Design review of the part built by this model. Coordinates are the model's own, in mm. A direction names the side the tool comes from. Round coordinates to 2 decimals unless told otherwise and drop trailing zeros. Write each loop counter-clockwise with the first axis right and the second up, starting at its lowest first coordinate (ties: lowest second). Pieces come first, ordered by that corner, then holes. Notation, with made-up numbers: (40, 65.25) -> (73, 65.25) arc R33 ccw to (73, 103.25) -> close; hole circle Ø7 at (74, 41.5). An arc over 180 degrees is marked (long way). Write item = value, one per line. Start each with the question number.
Item 1: For pin 1 Ø3 at (x, y) = (116, -31) entering from +Z; pin 2 Ø3 at (x, y) = (48, -29) entering from +Z; pin 3 Ø8 at (x, y) = (21, -20) entering from -Z, all flat-tipped, find the tip position at first contact; note any pin that passes through.
Item 2: Machinability: for faces 4 (the flat face through (48, -18, 6)), 5 (the flat face through (122, -27.059, 4)), 6 (the flat face through (50, -27.3, 4.5)), 7 (the flat face through (109, -30, 6)), 8 (the flat face through (3, -13, -13)), which of the approach directions +Z, -Z, +X, -X, +Y, -Y give a long, thin tool a straight path to every point of the face, cutting with its end or side? Answer none if there is none.
Item 3: Add section C-C, the plane x = 134.5. State the section outline as (y, z) points.
Item 4: Mouldability with a two-part tool opening along X and no side actions: class faces 1 (the flat face through (0, -13, -9)), 2 (the flat face through (113, -30, 5)), 3 (the flat face through (5, -23, 10)) as released by +X, released by -X, zero draft, split by the parting line, or undercut.
Item 5: Add section D-D, the plane y = -3. State the section outline as (x, z) points.
Item 6: Add section A-A, the plane y = -21. State the section outline as (x, z) points.
Item 7: To check wall thickness, follow L1, parallel to Z at x = 110.5, y = -30; L2, parallel to X at y = -17, z = -5; L3, parallel to Z at x = 68.5, y = -28.5. State the ranges of each line that lie inside material, in increasing order.
Item 8: Add section B-B, the plane z = 6.25. State how many separate pieces and enclosed holes the cut face has, then the cut area to 3 significant figures.
from build123d import *

# Parameters (mm, degrees)
SKETCH1_W           = 3
SKETCH1_H           = 20
BOSS_EXTRUDE1_DEPTH = 140
SKETCH3_W           = 10
SKETCH3_H           = 5.940571325
SKETCH3_W_2         = 4
SKETCH3_W_3         = 35
BOSS_EXTRUDE2_DEPTH = 10
SKETCH5_W           = 38
SKETCH5_H           = 5
CUT_EXTRUDE2_DEPTH  = 15
SKETCH6_W           = 10
SKETCH6_H           = 2.5
SKETCH6_W_2         = 4
BOSS_EXTRUDE4_DEPTH = 15
SKETCH7_R           = 1.75
SKETCH7_W           = 7.5
SKETCH7_H           = 2.5
CUT_EXTRUDE3_DEPTH  = 15
SKETCH9_W           = 20
SKETCH9_H           = 40
SKETCH9_R           = 2.25
BOSS_EXTRUDE5_DEPTH = 3
BOSS_EXTRUDE6_DEPTH = 3


with BuildPart() as part:
    # Sketch1 → Boss-Extrude1 (new body)
    with BuildSketch(Plane(origin=(0, 0, 0), x_dir=(0, 0, -1), z_dir=(1, 0, 0))):
        with Locations((1.5, -23)):
            Rectangle(SKETCH1_W, SKETCH1_H)
    extrude(amount=BOSS_EXTRUDE1_DEPTH)

    # Sketch3 → Boss-Extrude2 (add)
    with BuildSketch(Plane.XY):
        with Locations((5, -30.029714338)):
            Rectangle(SKETCH3_W, SKETCH3_H)
        with Locations((48, -30.029714338)):
            Rectangle(SKETCH3_W_2, SKETCH3_H)
        with Locations((82, -30.029714338)):
            Rectangle(SKETCH3_W_2, SKETCH3_H)
        with Locations((122.5, -30.029714338)):
            Rectangle(SKETCH3_W_3, SKETCH3_H)
    extrude(amount=BOSS_EXTRUDE2_DEPTH)

    # Sketch5 → Cut-Extrude2 (cut)
    with BuildSketch(Plane.XZ.offset(33)):
        with Locations((65, 7.5)):
            Rectangle(SKETCH5_W, SKETCH5_H)
    extrude(amount=-CUT_EXTRUDE2_DEPTH, mode=Mode.SUBTRACT)

    # Sketch6 → Boss-Extrude4 (add)
    with BuildSketch(Plane.XZ.offset(33)):
        with Locations((5, 11.25)):
            Rectangle(SKETCH6_W, SKETCH6_H)
        with Locations((48, 6.25)):
            Rectangle(SKETCH6_W_2, SKETCH6_H)
        with Locations((82, 6.25)):
            Rectangle(SKETCH6_W_2, SKETCH6_H)
    extrude(amount=-BOSS_EXTRUDE4_DEPTH)

    # Sketch7 → Cut-Extrude3 (cut)
    with BuildSketch(Plane(origin=(0, -27.059428675, 0), x_dir=(1, 0, 0), z_dir=(0, 1, 0))):
        with Locations((128.5, -6.25)):
            Circle(SKETCH7_R)
        with Locations((122.5, -6.25)):
            Circle(SKETCH7_R)
        with Locations((134.5, -6.25)):
            Circle(SKETCH7_R)
        with Locations((112.75, -6.25)):
            Rectangle(SKETCH7_W, SKETCH7_H)
    extrude(amount=-CUT_EXTRUDE3_DEPTH, mode=Mode.SUBTRACT)

    # Sketch9 → Boss-Extrude5 (add)
    with BuildSketch(Plane.ZY):
        with Locations((-13, -13)):
            Rectangle(SKETCH9_W, SKETCH9_H)
        with Locations((-13, -3)):
            Circle(SKETCH9_R, mode=Mode.SUBTRACT)
    extrude(amount=-BOSS_EXTRUDE5_DEPTH)

    # Sketch10 → Boss-Extrude6 (add)
    with BuildSketch(Plane.XY):
        Polygon((0, 7), (3, 7), (25, -13), (0, -13), align=None)
    extrude(amount=-BOSS_EXTRUDE6_DEPTH)


solid = part.part
Result set:
q1.pin_1 = 10
q1.pin_2 = 7.5
q1.pin_3 = -3
q2.face_4 = +Z, +X, -X, +Y
q2.face_5 = +Z, +X, +Y
q2.face_6 = +Z, +Y, -Y
q2.face_7 = +Y, -Y
q2.face_8 = -Z, +X, +Y, -Y
q3.outline = (-33, -3) -> (-13, -3) -> (-13, 0) -> (-27.06, 0) -> (-27.06, 4.5) -> (-33, 4.5) -> close; (-33, 8) -> (-27.06, 8) -> (-27.06, 10) -> (-33, 10) -> close
q4.face_1 = released by -X
q4.face_2 = undercut
q4.face_3 = zero draft
q5.outline = (0, -23) -> (3, -23) -> (3, -15.25) -> (0, -15.25) -> close; (0, -10.75) -> (3, -10.75) -> (3, -3) -> (14, -3) -> (14, 0) -> (0, 0) -> close
q6.outline = (0, -23) -> (3, -23) -> (3, -3) -> (140, -3) -> (140, 0) -> (0, 0) -> close; (0, 10) -> (10, 10) -> (10, 12.5) -> (0, 12.5) -> close; (46, 5) -> (50, 5) -> (50, 7.5) -> (46, 7.5) -> close; (80, 5) -> (84, 5) -> (84, 7.5) -> (80, 7.5) -> close
q7.L1 = -3 to 5, 7.5 to 10
q7.L2 = 0 to 3
q7.L3 = -3 to 0
q8.separate_pieces = 8
q8.enclosed_holes = 0
q8.area = 280 mm²
